Verification items for this drawing (mm, ordinates from the low corner). Coordinates: 2 decimals unless noted, no trailing zeros. Order: outer loops, then holes, each group sorted by start corner. A loop starts at its lowest first (then second) coordinate and runs counter-clockwise, first axis right, second up. Notation, with made-up numbers: (28, 66) -> (77, 66) arc R12 ccw to (77, 72) -> close; hole circle Ø11 at (-23.5, 6). An arc over 180 degrees is marked (long way). Answer in a Markdown table with one row per item. Add a question column.
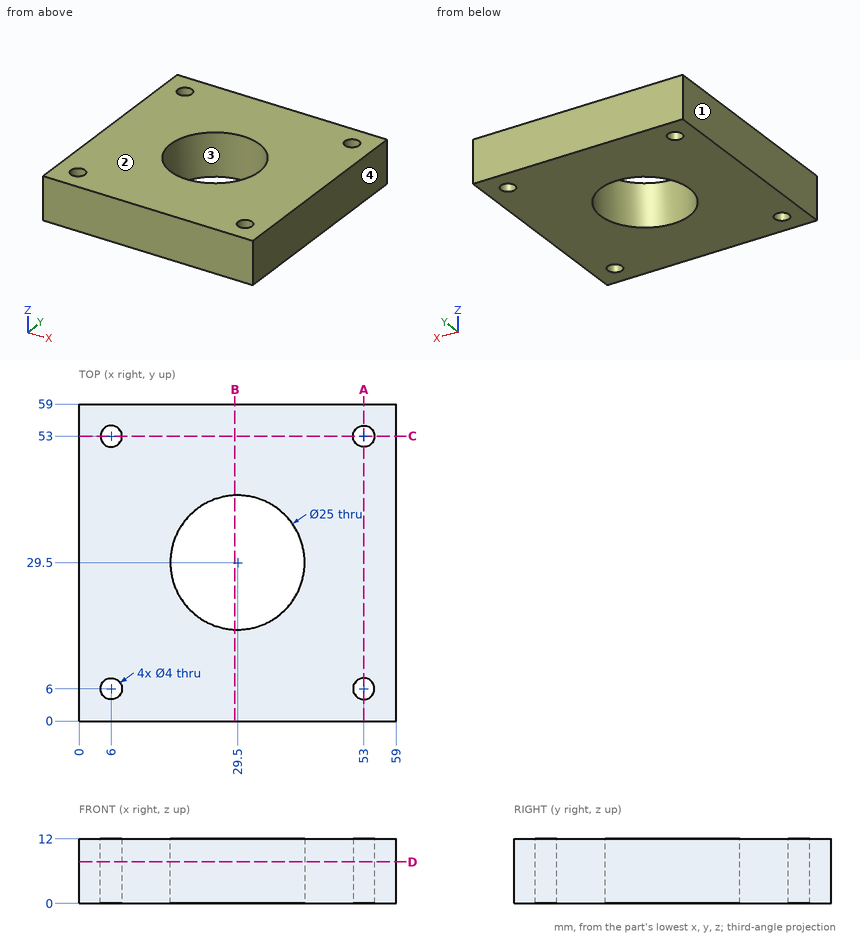
(1) Scan lines: line 1 along Y through (x, z) = (6, 6.25); line 2 along Y through (x, z) = (26, 3); line 3 along X through (y, z) = (18, 4.5). Record each from-to range of solid material in increasing order.
(2) Mould release check, pull along X, two halves, no side actions. Record for the marked faces 1, 2, 3 and 4: +X half, -X half, draft (parallel to the pull), parting line (faces both ways), or undercut.
(3) Cross-section at B-B (x = 29). Enter the section's corners in (y, z).
(4) Cross-section at D-D (z = 7.75). Enter the section's corners in (x, y).
(5) Cross-section at A-A (x = 53). Enter the section's corners in (y, z).
Checks:
| question | item | result |
|---|---|---|
| 1 | line 1 | 0 to 4, 8 to 51, 55 to 59 |
| 1 | line 2 | 0 to 17.5, 41.5 to 59 |
| 1 | line 3 | 0 to 24.6, 34.4 to 59 |
| 2 | face 1 | -X half |
| 2 | face 2 | draft |
| 2 | face 3 | undercut |
| 2 | face 4 | +X half |
| 3 | outline | (0, 0) -> (17.01, 0) -> (17.01, 12) -> (0, 12) -> close; (41.99, 0) -> (59, 0) -> (59, 12) -> (41.99, 12) -> close |
| 4 | outline | (0, 0) -> (59, 0) -> (59, 59) -> (0, 59) -> close; hole circle Ø4 at (6, 6); hole circle Ø4 at (6, 53); hole circle Ø25 at (29.5, 29.5); hole circle Ø4 at (53, 6); hole circle Ø4 at (53, 53) |
| 5 | outline | (0, 0) -> (4, 0) -> (4, 12) -> (0, 12) -> close; (8, 0) -> (51, 0) -> (51, 12) -> (8, 12) -> close; (55, 0) -> (59, 0) -> (59, 12) -> (55, 12) -> close |
